Could you check a few things on this model? Use its own coordinates, in mm. Face numbers are marked on the shaded views. Coordinates: 2 decimals unless noted, no trailing zeros. Write each loop counter-clockwise with the first axis right and the second up, starting at its lowest first coordinate (ties: lowest second). Pieces come first, ordered by that corner, then holes. Notation, with made-up numbers: M 41,60.5 L 100,60.5 A28 ccw 100,93.5 Z; hole C 7.25,71 d8. An arc over 180 degrees is marked long. Write item = value, one per line.
```python
from build123d import *

# Parameters (mm, degrees)
F0_W     = 152.4
F0_H     = 101.6
F1_DEPTH = 12.7
F2_R     = 3.81
F3_DEPTH = 25.4


# Not quite as in the source:
# - a feature names something its author has since deleted; it is built from what else it names


with BuildPart() as f1:
    # F0 (on Front) → F1 (new body)
    with BuildSketch(Plane.XZ):
        with Locations((76.2, 50.8)):
            Rectangle(F0_W, F0_H)
    extrude(amount=F1_DEPTH)

    # F2 (on face) → F3 (join)
    with BuildSketch(Plane.XZ.offset(12.7)):
        with Locations((14.4803142175, 12.5110410154)):
            Circle(F2_R)
        with Locations((14.4803142175, 37.9110410154)):
            Circle(F2_R)
        with Locations((14.4803142175, 63.3110410154)):
            Circle(F2_R)
        with Locations((14.4803142175, 88.7110410154)):
            Circle(F2_R)
        with Locations((39.8803142175, 12.5110410154)):
            Circle(F2_R)
        with Locations((39.8803142175, 37.9110410154)):
            Circle(F2_R)
        with Locations((39.8803142175, 63.3110410154)):
            Circle(F2_R)
        with Locations((39.8803142175, 88.7110410154)):
            Circle(F2_R)
        with Locations((65.2803142175, 12.5110410154)):
            Circle(F2_R)
        with Locations((65.2803142175, 37.9110410154)):
            Circle(F2_R)
        with Locations((65.2803142175, 63.3110410154)):
            Circle(F2_R)
        with Locations((65.2803142175, 88.7110410154)):
            Circle(F2_R)
        with Locations((90.6803142175, 12.5110410154)):
            Circle(F2_R)
        with Locations((90.6803142175, 37.9110410154)):
            Circle(F2_R)
        with Locations((90.6803142175, 63.3110410154)):
            Circle(F2_R)
        with Locations((90.6803142175, 88.7110410154)):
            Circle(F2_R)
        with Locations((116.0803142175, 12.5110410154)):
            Circle(F2_R)
        with Locations((116.0803142175, 37.9110410154)):
            Circle(F2_R)
        with Locations((116.0803142175, 63.3110410154)):
            Circle(F2_R)
        with Locations((116.0803142175, 88.7110410154)):
            Circle(F2_R)
        with Locations((141.4803142175, 12.5110410154)):
            Circle(F2_R)
        with Locations((141.4803142175, 37.9110410154)):
            Circle(F2_R)
        with Locations((141.4803142175, 63.3110410154)):
            Circle(F2_R)
        with Locations((141.4803142175, 88.7110410154)):
            Circle(F2_R)
    extrude(amount=F3_DEPTH)


solid = f1.part
```
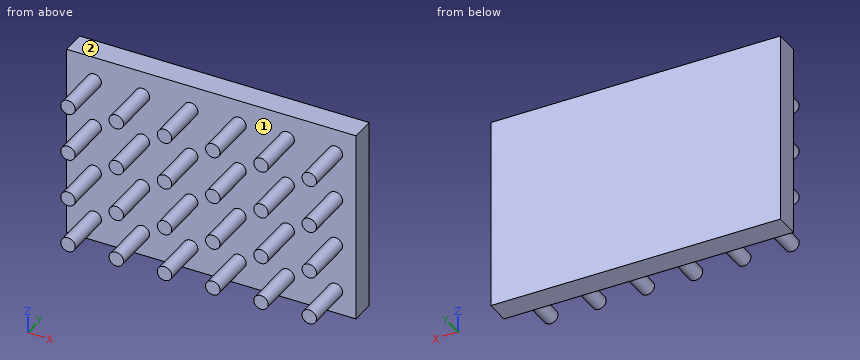
Item 1: Imagine slicing it at D-D (x = 124.5). Write out the boundary of the cut face in (y, z), and give its area (3 significant figures).
Numbers:
outline = M -12.7,0 L 0,0 L 0,101.6 L -12.7,101.6 Z
area = 1,290 mm²
Item 2: Imagine slicing it at A-A (y = -28.5). State how many separate pieces and enclosed holes the cut face has, and give its area (3 significant figures).
Numbers:
separate_pieces = 24
enclosed_holes = 0
area = 1,090 mm²
Item 3: Imagine slicing it at B-B (x = 15). Write out the boundary of the cut face in (y, z).
Numbers:
outline = M -38.1,8.74 L -12.7,8.74 L -12.7,0 L 0,0 L 0,101.6 L -12.7,101.6 L -12.7,92.49 L -38.1,92.49 L -38.1,84.94 L -12.7,84.94 L -12.7,67.09 L -38.1,67.09 L -38.1,59.54 L -12.7,59.54 L -12.7,41.69 L -38.1,41.69 L -38.1,34.14 L -12.7,34.14 L -12.7,16.29 L -38.1,16.29 Z
Item 4: I'm going to push a flat-ended pin straight in: P1, Ø3, axis at x = 103, z = 34.5, coming from the -Y side. Where does the tip first touch, or does it pass through?
Numbers:
P1 = -12.7
Item 5: If I drill on line 1 along Z through (x, y) = (14, -34.5); line 2 along X through (y, z) = (-19.5, 11.5); line 3 along Z through (x, y) = (39, -14), over which ranges is the centre line in solid material (lowest first)?
Numbers:
line_1 = 8.73 to 16.29, 34.13 to 41.69, 59.53 to 67.09, 84.93 to 92.49
line_2 = 10.81 to 18.15, 36.21 to 43.55, 61.61 to 68.95, 87.01 to 94.35, 112.41 to 119.75, 137.81 to 145.15
line_3 = 8.8 to 16.22, 34.2 to 41.62, 59.6 to 67.02, 85 to 92.42
Item 6: Imagine slicing it at C-C (z = 57). Write out the boundary of the cut face in (x, y).
Numbers:
outline = M 0,-12.7 L 152.4,-12.7 L 152.4,0 L 0,0 Z
Item 7: If we mould it in two halves opening along X, with no side actions, what happens to the marked faces 1 and 2? For each: pulls with the +X half, pulls with the -X half, needs draft (parallel to the pull), parting line crosses it, or undercut.
Numbers:
face_1 = undercut
face_2 = needs draft
